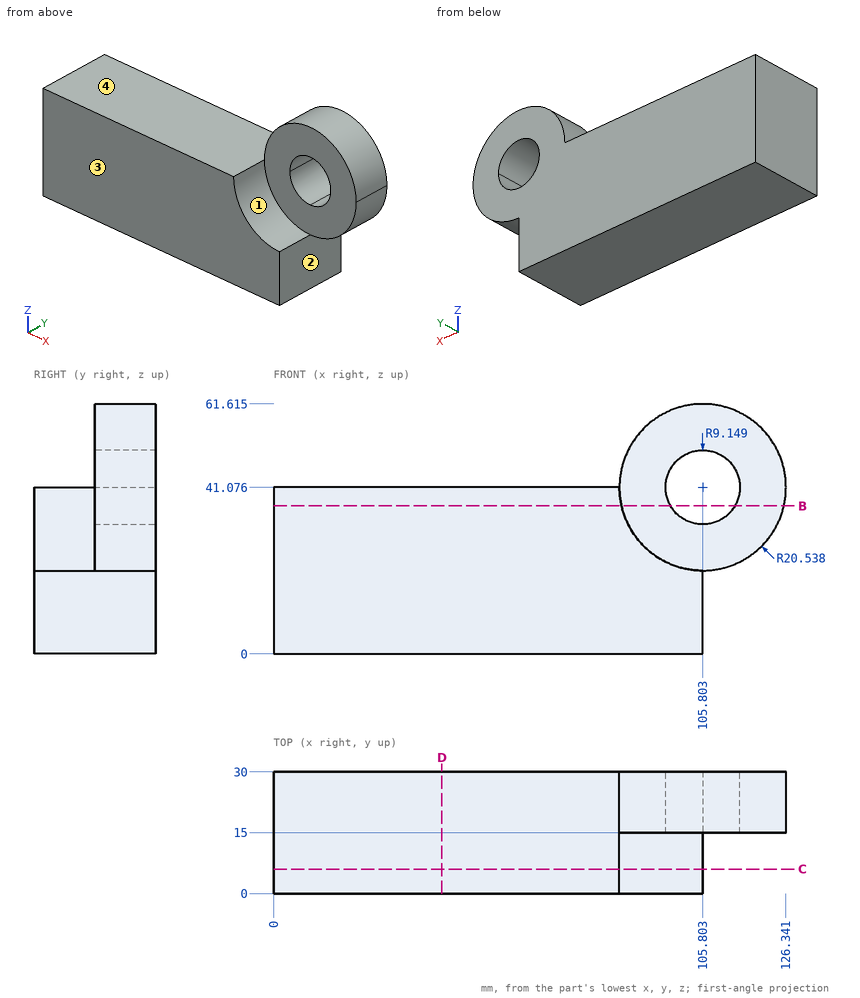
Print and shaded views of the part. All mm, measured from the part's lowest x, y and z. A direction names the side the tool comes from. Give positions to 0.01 mm unless a question says otherwise; leave off trailing zeros. Write each loop counter-clockwise with the first axis right and the second up, starting at its lowest first coordinate (ties: lowest second). Pieces come first, ordered by that corner, then holes. Notation, with made-up numbers: (21, 80) -> (55, 80) arc R15 cw to (55, 97) -> close; hole circle Ø1 at (2.5, 69.5). An arc over 180 degrees is marked (long way). Use CSV: the item, a comma, the result in double quotes. Start each with the question number.
1) Cut at D-D on x = 41.5. List the corners of the cut face in (y, z), plus the area to 3 significant figures.
2) Pin check, flat tips, straight feed: P1, Ø10, axis at x = 88.5, z = 51.5, coming from the -Y side; P2, Ø5, axis at x = 25, y = 26.5, coming from the +Z side. Stop position of each tip, or through.
3) Drill centre lines: L1, parallel to X at y = 10.5, z = 20.5; L2, parallel to Y at x = 114, z = 58; L3, parallel to Z at x = 12, y = 4.5. Where is each one in solid material? Low to high.
4) Cut at C-C on y = 6. List the corners of the cut face in (x, z) (1 decimal).
5) Cut at B-B on z = 36.5. List the corners of the cut face in (x, y) (1 decimal).
6) Tool access for the marked faces 1, 2, 3 and 4: list every direction of +Z, -Z, +X, -X, +Y, -Y with a clear straight run to the whole face (end or side of a thin tool).
Final values:
1,outline,"(0, 0) -> (30, 0) -> (30, 41.08) -> (0, 41.08) -> close"
1,area,"1,230 mm2"
2,P1,"stops at y = 15"
2,P2,"stops at z = 41.08"
3,L1,"x = 0 to 105.8"
3,L2,"y = 15 to 30"
3,L3,"z = 0 to 41.08"
4,outline,"(0, 0) -> (105.8, 0) -> (105.8, 20.5) arc R20.5 cw to (85.3, 41.1) -> (0, 41.1) -> close"
5,outline,"(0, 0) -> (85.8, 0) -> (85.8, 15) -> (97.9, 15) -> (97.9, 30) -> (0, 30) -> close; (113.7, 15) -> (125.8, 15) -> (125.8, 30) -> (113.7, 30) -> close"
6,face 1,"+Z, +X, -Y"
6,face 2,"-Z, +X, +Y, -Y"
6,face 3,"+Z, -Z, +X, -X, -Y"
6,face 4,"+Z, -X, +Y, -Y"
